```python
from build123d import *

# Parameters (mm, degrees)
F_3DSKETCH1_R         = 2.25
BOSS_EXTRUDE1_DEPTH   = 3.175
BOSS_EXTRUDE1_2_DEPTH = 3.175
BOSS_EXTRUDE1_3_DEPTH = 3.175
SKETCH2_W             = 3.175
SKETCH2_H             = 22.959761953
BOSS_EXTRUDE2_DEPTH   = 41.91
SKETCH3_W             = 67.66
SKETCH3_H             = 3.175
SKETCH3_W_2           = 7.05
BOSS_EXTRUDE3_DEPTH   = 7.62
SKETCH4_W             = 3.175
SKETCH4_H             = 30.579761953
BOSS_EXTRUDE4_DEPTH   = 4.318
CUT_EXTRUDE1_DEPTH    = 5.08
FILLET1_R             = 12.7


with BuildPart() as part:
    # 3DSketch1 → Boss-Extrude1 (new body)
    with BuildSketch(Plane(origin=(-464.25, 116.5, 0), x_dir=(-0.27427932364426477, -0.9616500676551969, 0), z_dir=(0, 0, -1))):
        Polygon((-1.923300135, 0.548558647), (0, 0), (18.333231377, 9.589323609), (19.93776542, 15.214976505), (99.754721035, -7.550207357), (98.150186992, -13.175860253), (108.666457645, -30.993563572), (110.58975778, -31.542122219), (117.652450364, -6.779632977), (5.139392449, 25.311047889), align=None)
        with Locations(Location((108.454058413, -17.154582881, 0), (0, 0, 254.080928829))):
            Circle(F_3DSKETCH1_R, mode=Mode.SUBTRACT)
        with Locations(Location((7.480801309, 11.644746102, 0), (0, 0, 254.080928829))):
            Circle(F_3DSKETCH1_R, mode=Mode.SUBTRACT)
    extrude(amount=-BOSS_EXTRUDE1_DEPTH)



with BuildPart() as body_2:
    # 3DSketch1 → Boss-Extrude1 2 (new body)
    with BuildSketch(Plane(origin=(-464.25, 116.5, 0), x_dir=(-0.27427932364426477, -0.9616500676551969, 0), z_dir=(0, 0, -1))):
        Polygon((-24.002556771, 6.845946627), (-1.923300135, 0.548558647), (5.139392449, 25.311047889), (-16.939864187, 31.608435869), align=None)
    extrude(amount=-BOSS_EXTRUDE1_2_DEPTH)


with BuildPart() as body_3:
    # 3DSketch1 → Boss-Extrude1 3 (new body)
    with BuildSketch(Plane(origin=(-464.25, 116.5, 0), x_dir=(-0.27427932364426477, -0.9616500676551969, 0), z_dir=(0, 0, -1))):
        Polygon((-16.939864187, 31.608435869), (5.139392449, 25.311047889), (117.652450364, -6.779632977), (119.586119596, 0), (-15.006194955, 38.388068846), align=None)
    extrude(amount=-BOSS_EXTRUDE1_3_DEPTH)


with BuildPart() as part_1:
    add(part.part)

    add(body_2.part)  # Boss-Extrude2 merges body 2
    # Sketch2 → Boss-Extrude2 (add)
    with BuildSketch(Plane(origin=(-464.25, 0, 0), x_dir=(0, 0, -1), z_dir=(1, 0, 0))):
        with Locations((-1.5875, 129.979880976)):
            Rectangle(SKETCH2_W, SKETCH2_H)
    extrude(amount=BOSS_EXTRUDE2_DEPTH)


    add(body_3.part)  # Boss-Extrude3 merges body 3
    # Sketch3 → Boss-Extrude3 (add)
    with BuildSketch(Plane(origin=(0, 141.459761953, 0), x_dir=(1, 0, 0), z_dir=(0, 1, 0))):
        with Locations((-456.17, -1.5875)):
            Rectangle(SKETCH3_W, SKETCH3_H)
        with Locations((-493.525, -1.5875)):
            Rectangle(SKETCH3_W_2, SKETCH3_H)
    extrude(amount=BOSS_EXTRUDE3_DEPTH)

    # Sketch4 → Boss-Extrude4 (add)
    with BuildSketch(Plane(origin=(-422.34, 0, 0), x_dir=(0, 0, -1), z_dir=(1, 0, 0))):
        with Locations((-1.5875, 133.789880977)):
            Rectangle(SKETCH4_W, SKETCH4_H)
    extrude(amount=BOSS_EXTRUDE4_DEPTH)

    # Sketch5 → Cut-Extrude1 (cut)
    with BuildSketch(Plane.XY.offset(3.175)):
        with BuildLine():
            Line((-426.539082165, 149.079761953), (-418.022, 149.079761953))
            Line((-418.022, 149.079761953), (-418.022, 126.606320753))
            add(Edge.make_bspline(
                [(-418.022, 126.606320753), (-422.206786757, 127.841281747), (-432.70768746, 132.592685738), (-432.363764658, 146.022941569), (-426.539082165, 149.079761953)],
                knots=[0, 0, 0, 0, 0.445070819, 1, 1, 1, 1], degree=3))
        make_face()
        Polygon((-497.05, 118.5), (-464.25, 149.079761953), (-497.05, 149.079761953), align=None)
    extrude(amount=-CUT_EXTRUDE1_DEPTH, mode=Mode.SUBTRACT)

    # Fillet1
    fillet1_edges = [part_1.edges().sort_by_distance(p)[0] for p in [
        (-497.05, 1.5, 1.5875),
        (-464.25, 149.079761953, 1.5875),
        (-497.05, 118.5, 1.5875),
    ]]
    fillet(fillet1_edges, radius=FILLET1_R)


solid = part_1.part
```
Geometry: final body of the model. Coordinates: model frame, mm. A direction names the side the tool comes from. Round coordinates to 2 decimals unless told otherwise and drop trailing zeros. Order: outer loops, then holes, each group sorted by start corner. A loop starts at its lowest first (then second) coordinate and runs counter-clockwise, first axis right, second up. Notation, with made-up numbers: M 23.5,54 L 55.5,54 A6 cw 55.5,59 Z; hole C -6.75,49.25 d9. An arc over 180 degrees is marked long. Use one line per item in the form item = value. Start each with the question number.
Q1. Cut plane C-C (y = 57). Return loops of the section in (x, z) (3 decimals), and give its area (3 significant figures).
Q2. Pin query (flat end, axial travel): pin 1 Ø1 at (x, z) = (-483, 1) entering from +Y; pin 2 Ø1.6 at (y, z) = (2.5, 2) entering from +X; pin 3 Ø5 at (x, y) = (-477.5, 7.5) entering from +Z (3 decimals); pin 4 Ø1.6 at (x, z) = (-482, 2) entering from +Y. Return the tip coordinate at first contact, or that it passes through.
Q3. Access query for faces 1 (the face through (-441, 118.5, 2)), 2 (the face through (-443, 149.08, 2)), 3 (the face through (-481, 18.5, 2)). Directions: +Z, -Z, +X, -X, +Y, -Y. A direction counts if a zero-diameter tool reaches every point of the face in a straight line with its end or side. Return the directions, or none.
Q4. Mould query, pull axis X, two halves, no side actions, for faces 4 (the face through (-478.2, 102.3, 3.175)), 5 (the face through (-471.475, 11.105, 1.565)), 6 (the face through (-496.025, 117.975, 1.565)), 7 (the face through (-479.748, 112.401, 1.565)). Classes: +X half, -X half, draft (parallel to the pull), parting line (faces both ways), or undercut.
Q5. Cut plane A-A (x = -482). Return loops of the section in (y, z) (3 decimals).
Q6. Cut plane B-B (z = 1.55). Count the separate pieces of the cut face and the enclosed holes in it, and give its area (3 significant figures).
Q7. Cut plane D-D (x = -457.5). Return loops of the section in (y, z) (3 decimals), and give its area (3 significant figures).
Q8. Material intervals for line 1 (Y direction, x = -477.5, z = 2.1); line 2 (X direction, y = 43, z = 2.5), sorted ascending. Write a range as [from, to].
Geometry results:
q1.outline = M -497.05,0 L -484.35,0 L -484.35,3.175 L -497.05,3.175 Z
q1.area = 40.3 mm^2
q2.pin_1 = 132.07
q2.pin_2 = -464.25
q2.pin_3 = 3.175
q2.pin_4 = 133.28
q3.face_1 = +Z, -Z, +X, -Y
q3.face_2 = +Z, -Z, +X, -X, +Y
q3.face_3 = +Z, -Z, +X
q4.face_4 = draft
q4.face_5 = +X half
q4.face_6 = -X half
q4.face_7 = undercut
q5.outline = M 1.5,0 L 18.5,0 L 18.5,3.175 L 1.5,3.175 Z; M 101.5,0 L 132.531,0 L 132.531,3.175 L 101.5,3.175 Z
q6.separate_pieces = 1
q6.enclosed_holes = 2
q6.area = 3,560 mm^2
q7.outline = M 118.5,0 L 149.08,0 L 149.08,3.175 L 118.5,3.175 Z
q7.area = 97.1 mm^2
q8.line_1 = [1.5, 5.25], [9.75, 17.45], [102.55, 110.25], [114.75, 136.73]
q8.line_2 = [-497.05, -484.35]
